```python
from build123d import *

# Parameters (mm, degrees)
BOSS_EXTRU_1_DEPTH      = 3
BOSS_EXTRU_1_DEPTH_BACK = 3
ESQUISSE1_R             = 2
ESQUISSE2_W             = 10
ESQUISSE2_H             = 11.041575451
ENL_V_MAT_EXTRU_1_DEPTH = 3


with BuildPart() as part:
    # Esquisse1 → Boss.-Extru.1 (new, two sides: drawn at the far end of the back side and taken through both)
    with BuildSketch(Plane(origin=(0, 0, 0), x_dir=(1, 0, 0), z_dir=(0, 1, 0)).offset(-BOSS_EXTRU_1_DEPTH_BACK)):
        with BuildLine():
            Line((-5, -40), (-5, 0))
            ThreePointArc((-5, 0), (0, 5), (5, 0))
            Line((5, 0), (5, -40))
            ThreePointArc((5, -40), (0, -45), (-5, -40))
        make_face()
        with Locations(Location((0, 0, 0), (0, 0, 270))):
            Circle(ESQUISSE1_R, mode=Mode.SUBTRACT)
        with Locations(Location((0, -40, 0), (0, 0, 270))):
            Circle(ESQUISSE1_R, mode=Mode.SUBTRACT)
    extrude(amount=BOSS_EXTRU_1_DEPTH + BOSS_EXTRU_1_DEPTH_BACK)

    # Esquisse2 → Enl_v. mat.-Extru.1 (cut)
    with BuildSketch(Plane(origin=(0, 3, 0), x_dir=(1, 0, 0), z_dir=(0, 1, 0))):
        with Locations((0, -40.520787725)):
            Rectangle(ESQUISSE2_W, ESQUISSE2_H)
    extrude(amount=-ENL_V_MAT_EXTRU_1_DEPTH, mode=Mode.SUBTRACT)


solid = part.part
```
Check sheet for the modelled part. Datum: model origin and axes. Units: mm. A direction names the side the tool comes from. Give positions to 0.01 mm unless a question says otherwise; leave off trailing zeros. Order: outer loops, then holes, each group sorted by start corner. A loop starts at its lowest first (then second) coordinate and runs counter-clockwise, first axis right, second up. Notation, with made-up numbers: M 86.5,-14 L 139.5,-14 A17 ccw 139.5,10 Z; hole C 13,64.25 d3. An arc over 180 degrees is marked long. Answer in a Markdown table with one row per item. Add a question column.
Q1. Access from +Z, -Z, +X, -X, +Y, -Y to the whole of each face (thin tool, end or side, straight path). Record for faces 5 (the flat face through (-0.1, 0, 37.7)), 6 (the flat face through (0, 3, 15)).
Q2. Release check for a two-part mould opening along X. For faces 1 (the cylindrical face through (-2, 0, 0)), 2 (the cylindrical face through (0, -2, 38)), 3 (the flat face through (0, -3, 20)), 4 (the flat face through (-5, 0, 20)) record: released by +X, released by -X, zero draft, split by the parting line, or undercut.
Q3. Gauge pin test, flat ends, axial feed: pin 1 Ø1.5 at (x, y) = (3, -2) entering from +Z; pin 2 Ø3 at (x, y) = (2, -2) entering from +Z; pin 3 Ø1.5 at (x, y) = (-1.5, 1) entering from +Z. Record the tip position at first contact, or that the pin passes through.
Q4. Sectioned sample at D-D, the plane x = -3. Record the boundary of the cut face in (y, z), and give its area (3 significant figures).
Q5. Sectioned sample at C-C, the plane z = 41.5. Record the boundary of the cut face in (x, y), and give its area (3 significant figures).
Q6. Sectioned sample at A-A, the plane x = 0. Record the boundary of the cut face in (y, z), and give its area (3 significant figures).
Q7. Thickness scan on L1, parallel to X at y = -0.8, z = 40; L2, parallel to Z at x = -0.5, y = -1.5; L3, parallel to Z at x = 1.5, y = -2.05. Record the ranges inside material, lowest first.
Q8. Sectioned sample at B-B, the plane y = -1.5. Record the boundary of the cut face in (x, z).
Verdict:
| question | item | result |
|---|---|---|
| 1 | face 5 | +Z, +X, -X, +Y |
| 1 | face 6 | +Z, -Z, +X, -X, +Y |
| 2 | face 1 | undercut |
| 2 | face 2 | undercut |
| 2 | face 3 | zero draft |
| 2 | face 4 | released by -X |
| 3 | pin 1 | z = 44.47 |
| 3 | pin 2 | z = 44.97 |
| 3 | pin 3 | z = 35 |
| 4 | outline | M -3,-4 L 3,-4 L 3,35 L 0,35 L 0,44 L -3,44 Z |
| 4 | area | 261 mm² |
| 5 | outline | M -4.77,-3 L -1.32,-3 L -1.32,0 L -4.77,0 Z; M 1.32,-3 L 4.77,-3 L 4.77,0 L 1.32,0 Z |
| 5 | area | 20.7 mm² |
| 6 | outline | M -3,-5 L 3,-5 L 3,-2 L -3,-2 Z; M -3,2 L 3,2 L 3,35 L 0,35 L 0,38 L -3,38 Z; M -3,42 L 0,42 L 0,45 L -3,45 Z |
| 6 | area | 234 mm² |
| 7 | L1 | -5 to -2, 2 to 5 |
| 7 | L2 | -4.97 to -1.94, 1.94 to 38.06, 41.94 to 44.97 |
| 7 | L3 | -4.77 to -1.32, 1.32 to 38.68, 41.32 to 44.77 |
| 8 | outline | M -5,0 A5 ccw 5,0 L 5,40 A5 ccw -5,40 Z; hole C 0,0 d4; hole C 0,40 d4 |
